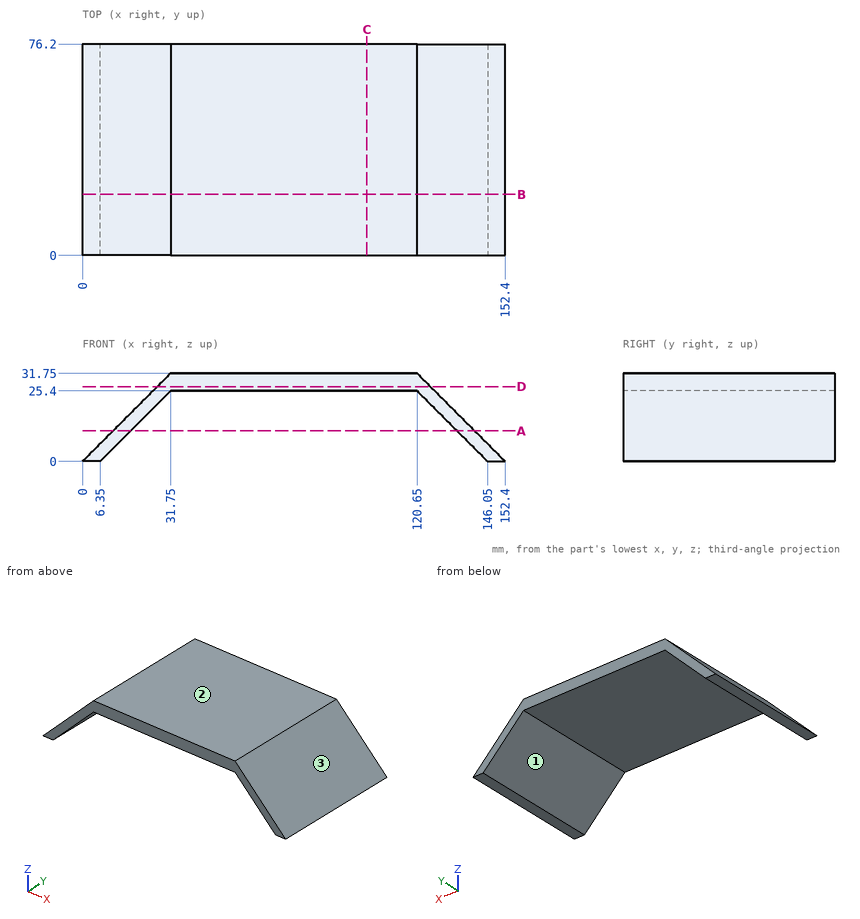
Print and shaded views of the part. All mm, measured from the part's lowest x, y and z. Give positions to 0.01 mm unless a question says otherwise; leave off trailing zeros. Order: outer loops, then holes, each group sorted by start corner. A loop starts at its lowest first (then second) coordinate and runs counter-clockwise, first axis right, second up. Notation, with made-up numbers: (62.5, 61) - (104.5, 61) arc R14 ccw to (104.5, 72) - close; hole circle Ø11 at (-15.5, -18.5). An arc over 180 degrees is marked (long way). One line per item, written item: value.
Item 1: Pin check, flat tips, straight feed: pin 1 Ø6 at (y, z) = (9, 23) entering from +X; pin 2 Ø1.5 at (y, z) = (36.5, 26) entering from +X; pin 3 Ø8 at (x, y) = (132.5, 23.5) entering from -Z. Stop position of each tip, or through.
Response values:
pin 1: x = 132.4
pin 2: x = 127.15
pin 3: z = 9.55
Item 2: Slice it at A-A (z = 11). List the corners of the cut face in (x, y), then the cut area to 3 significant figures.
Response values:
outline: (11, 0) - (17.35, 0) - (17.35, 76.2) - (11, 76.2) - close; (135.05, 0) - (141.4, 0) - (141.4, 76.2) - (135.05, 76.2) - close
area: 968 mm2
Item 3: Slice it at D-D (z = 27). List the corners of the cut face in (x, y).
Response values:
outline: (27, 0) - (125.4, 0) - (125.4, 76.2) - (27, 76.2) - close
Item 4: Two-plate mould, pull along X, no slides. Class the marked faces 1, 2 and 3: released by +X, released by -X, zero draft, split by the parting line, or undercut.
Response values:
face 1: undercut
face 2: zero draft
face 3: released by +X
Item 5: Slice it at B-B (y = 22). List the corners of the cut face in (x, z), then the cut area to 3 significant figures.
Response values:
outline: (0, 0) - (6.35, 0) - (31.75, 25.4) - (120.65, 25.4) - (146.05, 0) - (152.4, 0) - (120.65, 31.75) - (31.75, 31.75) - close
area: 927 mm2
Item 6: Wall check: line 1 (Z direction, x = 94, y = 45); line 2 (X direction, y = 40, z = 14); line 3 (X direction, y = 46.5, z = 7). Give the ranges that are in metal, low to high.
Response values:
line 1: 25.4 to 31.75
line 2: 14 to 20.35, 132.05 to 138.4
line 3: 7 to 13.35, 139.05 to 145.4
Item 7: Slice it at C-C (x = 102.5). List the corners of the cut face in (y, z).
Response values:
outline: (0, 25.4) - (76.2, 25.4) - (76.2, 31.75) - (0, 31.75) - close
